Verification items for the finished model (mm, model axes). Face numbers are marked on the shaded views. A direction names the side the tool comes from. Give positions to 0.01 mm unless a question says otherwise; leave off trailing zeros. Put each result on its own line as item: value. Start each with the question number.
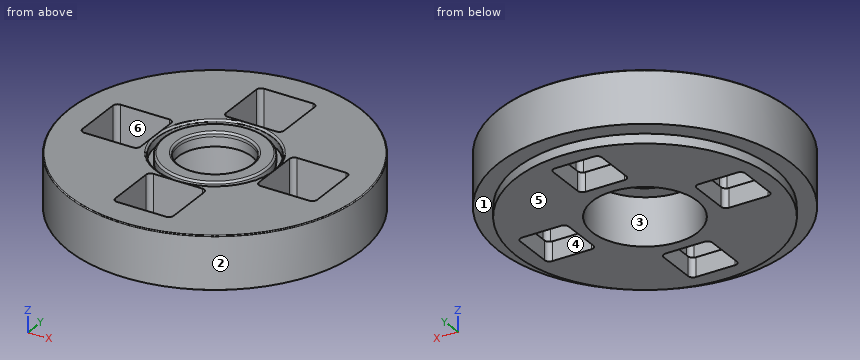
from build123d import *

# Parameters (mm, degrees)
IZIM1_R                     = 135
Y_KSEKLIK_EKSTR_ZYON1_DEPTH = 60
Y_KSEKLIK_EKSTR_ZYON2_START = 10
IZIM2_R                     = 153
Y_KSEKLIK_EKSTR_ZYON2_DEPTH = 50
IZIM3_R                     = 55
KES_EKSTR_ZYON1_DEPTH       = 741
Y_KSEKLIK_EKSTR_ZYON3_START = -50
IZIM4_R                     = 55
IZIM4_R_2                   = 38.5
Y_KSEKLIK_EKSTR_ZYON3_DEPTH = 10
IZIM5_R                     = 153
IZIM5_R_2                   = 38.5
Y_KSEKLIK_EKSTR_ZYON4_DEPTH = 5
IZIM6_R                     = 60.5
IZIM6_R_2                   = 54.5
KES_EKSTR_ZYON2_DEPTH       = 10
RADYUS2_R                   = 2
FILLET1_R                   = 1
CUT_EXTRUDE1_START          = -20
CUT_EXTRUDE1_DEPTH          = 206.926979422
CUT_EXTRUDE2_DEPTH          = 226.92697945


with BuildPart() as part:
    # Çizim1 → Yükseklik-Ekstrüzyon1 (new body)
    with BuildSketch(Plane.XY):
        Circle(IZIM1_R)
    extrude(amount=Y_KSEKLIK_EKSTR_ZYON1_DEPTH)

    # Çizim2 → Yükseklik-Ekstrüzyon2 (add)
    with BuildSketch(Plane.XY.offset(Y_KSEKLIK_EKSTR_ZYON2_START)):
        Circle(IZIM2_R)
    extrude(amount=Y_KSEKLIK_EKSTR_ZYON2_DEPTH)

    # Çizim3 → Kes-Ekstrüzyon1 (cut)
    with BuildSketch(Plane(origin=(0, 0, 0), x_dir=(-1, 0, 0), z_dir=(0, 0, -1))):
        Circle(IZIM3_R)
    extrude(amount=-KES_EKSTR_ZYON1_DEPTH, mode=Mode.SUBTRACT)

    # Çizim4 → Yükseklik-Ekstrüzyon3 (add)
    with BuildSketch(Plane(origin=(0, 0, 0), x_dir=(-1, 0, 0), z_dir=(0, 0, -1)).offset(Y_KSEKLIK_EKSTR_ZYON3_START)):
        Circle(IZIM4_R)
        Circle(IZIM4_R_2, mode=Mode.SUBTRACT)
    extrude(amount=-Y_KSEKLIK_EKSTR_ZYON3_DEPTH)

    # Çizim5 → Yükseklik-Ekstrüzyon4 (add)
    with BuildSketch(Plane.XY.offset(60)):
        Circle(IZIM5_R)
        with Locations(Location((0, 0, 0), (0, 0, 180))):
            Circle(IZIM5_R_2, mode=Mode.SUBTRACT)
    extrude(amount=Y_KSEKLIK_EKSTR_ZYON4_DEPTH)

    # Çizim6 → Kes-Ekstrüzyon2 (cut)
    with BuildSketch(Plane.XY.offset(65)):
        Circle(IZIM6_R)
        Circle(IZIM6_R_2, mode=Mode.SUBTRACT)
    extrude(amount=-KES_EKSTR_ZYON2_DEPTH, mode=Mode.SUBTRACT)

    # Radyus2
    radyus2_edges = [part.edges().sort_by_distance(p)[0] for p in [
        (38.5, 0, 65),
        (-60.5, 0, 65),
        (-54.5, 0, 65),
    ]]
    fillet(radyus2_edges, radius=RADYUS2_R)

    # Fillet1
    fillet1_edges = [part.edges().sort_by_distance(p)[0] for p in [
        (-153, 0, 65),
    ]]
    fillet(fillet1_edges, radius=FILLET1_R)

    # Sketch1 → Cut-Extrude1 (cut, through all)
    with BuildSketch(Plane(origin=(0, 0, 0), x_dir=(-1, 0, 0), z_dir=(0, 0, -1)).offset(CUT_EXTRUDE1_START)):
        with BuildLine():
            Line((25.5, 123), (-25.5, 123))
            ThreePointArc((-25.5, 123), (-29.035533906, 121.535533906), (-30.5, 118))
            Line((-30.5, 118), (-30.5, 67))
            ThreePointArc((-30.5, 67), (-29.035533906, 63.464466094), (-25.5, 62))
            Line((-25.5, 62), (25.5, 62))
            ThreePointArc((25.5, 62), (29.035533906, 63.464466094), (30.5, 67))
            Line((30.5, 67), (30.5, 118))
            ThreePointArc((30.5, 118), (29.035533906, 121.535533906), (25.5, 123))
        make_face()
        with BuildLine():
            Line((-118, 30.5), (-67, 30.5))
            ThreePointArc((-67, 30.5), (-63.464466094, 29.035533906), (-62, 25.5))
            Line((-62, 25.5), (-62, -25.5))
            ThreePointArc((-62, -25.5), (-63.464466094, -29.035533906), (-67, -30.5))
            Line((-67, -30.5), (-118, -30.5))
            ThreePointArc((-118, -30.5), (-121.535533906, -29.035533906), (-123, -25.5))
            Line((-123, -25.5), (-123, 25.5))
            ThreePointArc((-123, 25.5), (-121.535533906, 29.035533906), (-118, 30.5))
        make_face()
        with BuildLine():
            Line((123, -25.5), (123, 25.5))
            ThreePointArc((123, 25.5), (121.535533906, 29.035533906), (118, 30.5))
            Line((118, 30.5), (67, 30.5))
            ThreePointArc((67, 30.5), (63.464466094, 29.035533906), (62, 25.5))
            Line((62, 25.5), (62, -25.5))
            ThreePointArc((62, -25.5), (63.464466094, -29.035533906), (67, -30.5))
            Line((67, -30.5), (118, -30.5))
            ThreePointArc((118, -30.5), (121.535533906, -29.035533906), (123, -25.5))
        make_face()
        with BuildLine():
            Line((-25.5, -123), (25.5, -123))
            ThreePointArc((25.5, -123), (29.035533906, -121.535533906), (30.5, -118))
            Line((30.5, -118), (30.5, -67))
            ThreePointArc((30.5, -67), (29.035533906, -63.464466094), (25.5, -62))
            Line((25.5, -62), (-25.5, -62))
            ThreePointArc((-25.5, -62), (-29.035533906, -63.464466094), (-30.5, -67))
            Line((-30.5, -67), (-30.5, -118))
            ThreePointArc((-30.5, -118), (-29.035533906, -121.535533906), (-25.5, -123))
        make_face()
    extrude(amount=-CUT_EXTRUDE1_DEPTH, mode=Mode.SUBTRACT)

    # Sketch2 → Cut-Extrude2 (cut, through all)
    with BuildSketch(Plane(origin=(0, 0, 0), x_dir=(-1, 0, 0), z_dir=(0, 0, -1))):
        with BuildLine():
            Line((20.5, 118), (-20.5, 118))
            ThreePointArc((-20.5, 118), (-24.035533906, 116.535533906), (-25.5, 113))
            Line((-25.5, 113), (-25.5, 72))
            ThreePointArc((-25.5, 72), (-24.035533906, 68.464466094), (-20.5, 67))
            Line((-20.5, 67), (20.5, 67))
            ThreePointArc((20.5, 67), (24.035533906, 68.464466094), (25.5, 72))
            Line((25.5, 72), (25.5, 113))
            ThreePointArc((25.5, 113), (24.035533906, 116.535533906), (20.5, 118))
        make_face()
        with BuildLine():
            Line((-113, 25.5), (-72, 25.5))
            ThreePointArc((-72, 25.5), (-68.464466094, 24.035533906), (-67, 20.5))
            Line((-67, 20.5), (-67, -20.5))
            ThreePointArc((-67, -20.5), (-68.464466094, -24.035533906), (-72, -25.5))
            Line((-72, -25.5), (-113, -25.5))
            ThreePointArc((-113, -25.5), (-116.535533906, -24.035533906), (-118, -20.5))
            Line((-118, -20.5), (-118, 20.5))
            ThreePointArc((-118, 20.5), (-116.535533906, 24.035533906), (-113, 25.5))
        make_face()
        with BuildLine():
            Line((118, -20.5), (118, 20.5))
            ThreePointArc((118, 20.5), (116.535533906, 24.035533906), (113, 25.5))
            Line((113, 25.5), (72, 25.5))
            ThreePointArc((72, 25.5), (68.464466094, 24.035533906), (67, 20.5))
            Line((67, 20.5), (67, -20.5))
            ThreePointArc((67, -20.5), (68.464466094, -24.035533906), (72, -25.5))
            Line((72, -25.5), (113, -25.5))
            ThreePointArc((113, -25.5), (116.535533906, -24.035533906), (118, -20.5))
        make_face()
        with BuildLine():
            Line((-20.5, -118), (20.5, -118))
            ThreePointArc((20.5, -118), (24.035533906, -116.535533906), (25.5, -113))
            Line((25.5, -113), (25.5, -72))
            ThreePointArc((25.5, -72), (24.035533906, -68.464466094), (20.5, -67))
            Line((20.5, -67), (-20.5, -67))
            ThreePointArc((-20.5, -67), (-24.035533906, -68.464466094), (-25.5, -72))
            Line((-25.5, -72), (-25.5, -113))
            ThreePointArc((-25.5, -113), (-24.035533906, -116.535533906), (-20.5, -118))
        make_face()
    extrude(amount=-CUT_EXTRUDE2_DEPTH, mode=Mode.SUBTRACT)


solid = part.part
Q1. Scan lines: L1, parallel to Y at x = 0, z = 61; L2, parallel to Y at x = 18.5, z = 13; L3, parallel to X at y = 11.5, z = 29.5. Record each from-to range of solid material in increasing order.
Q2. Release check for a two-part mould opening along X. For the marked faces 1, 2 and 3 record: pulls with the +X half, pulls with the -X half, needs draft (parallel to the pull), parting line crosses it, or undercut.
Q3. Cross-section at A-A, the plane z = 40. State how many separate pieces and enclosed holes the cut face has, then the cut area to 3 significant figures.
Q4. Go/stop test with flat-tipped pins: pin 1 (3 mm diameter, centred on x = 104.5, z = 25, fed in from +Y); pin 2 (13.5 mm diameter, centred on x = -96.5, z = 44, fed in from +Y); pin 3 (1.5 mm diameter, centred on x = 61.5, z = 44, fed in from -Y); pin 4 (1.5 mm diameter, centred on x = 60, y = -120, fed in from -Z). Record where each tip stops, or that it passes through.
Q5. Set-up check for the marked faces 4, 5 and 6: record each of +Z, -Z, +X, -X, +Y, -Y from which the full face is reachable in a straight line by a thin tool's end or side.
Ans:
1. L1: y = -153 to -123, -62 to -60.5, -54.5 to -38.5, 38.5 to 54.5, 60.5 to 62, 123 to 153
1. L2: y = -151.88 to -118, -67 to -51.8, 51.8 to 67, 118 to 151.88
1. L3: x = -152.57 to -123, -62 to -53.78, 53.78 to 62, 123 to 152.57
2. face 1: needs draft
2. face 2: parting line crosses it
2. face 3: undercut
3. separate pieces: 1
3. enclosed holes: 5
3. area: 49,200 mm^2
4. pin 1: stops at y = 113.14
4. pin 2: stops at y = 123.91
4. pin 3: stops at y = -140.42
4. pin 4: stops at z = 0
5. face 4: +Z, -Z
5. face 5: -Z, +X, -X, +Y, -Y
5. face 6: +Z
